Work out the finished part from the listing and answer in its coordinate system (mm). A direction names the side the tool comes from. Round coordinates to 2 decimals unless told otherwise and drop trailing zeros. Loops run counter-clockwise (first coordinate to the right, second up) from the corner with the lowest first, then second, coordinate; pieces in that order, holes last. Notation, with made-up numbers: (81.25, 17) -> (117.25, 17) arc R8 ccw to (117.25, 27) -> close; hole circle Ø7 at (-19.75, 47). An arc over 180 degrees is marked (long way). Use one line per item in the form item = value.
```python
from build123d import *

# Parameters (mm, degrees)
SKETCH2_R           = 1.95
SKETCH2_R_2         = 12.5
BOSS_EXTRUDE1_DEPTH = 3.175


with BuildPart() as part:
    # Sketch2 → Boss-Extrude1 (new body)
    with BuildSketch(Plane.XY):
        Polygon((-3.175, 0), (66.675, 0), (66.675, 12.7), (63.5, 12.7), (63.5, 14.375), (60.412, 14.375), (60.412, 12.625), (57.912, 12.625), (57.912, 14.375), (57.15, 14.375), (57.15, 17.375), (57.912, 17.375), (57.912, 19.125), (60.412, 19.125), (60.412, 17.375), (63.5, 17.375), (63.5, 27.075), (60.412, 27.075), (60.412, 25.325), (57.912, 25.325), (57.912, 27.075), (57.15, 27.075), (57.15, 30.075), (57.912, 30.075), (57.912, 31.825), (60.412, 31.825), (60.412, 30.075), (63.5, 30.075), (63.5, 31.75), (66.675, 31.75), (66.675, 44.45), (-3.175, 44.45), (-3.175, 31.75), (0, 31.75), (0, 30.075), (3.088, 30.075), (3.088, 31.825), (5.588, 31.825), (5.588, 30.075), (6.35, 30.075), (6.35, 27.075), (5.588, 27.075), (5.588, 25.325), (3.088, 25.325), (3.088, 27.075), (0, 27.075), (0, 17.375), (3.088, 17.375), (3.088, 19.125), (5.588, 19.125), (5.588, 17.375), (6.35, 17.375), (6.35, 14.375), (5.588, 14.375), (5.588, 12.625), (3.088, 12.625), (3.088, 14.375), (0, 14.375), (0, 12.7), (-3.175, 12.7), align=None)
        with Locations((16.25, 6.725)):
            Circle(SKETCH2_R, mode=Mode.SUBTRACT)
        with Locations((47.25, 6.725)):
            Circle(SKETCH2_R, mode=Mode.SUBTRACT)
        with Locations((16.25, 37.725)):
            Circle(SKETCH2_R, mode=Mode.SUBTRACT)
        with Locations((31.75, 22.225)):
            Circle(SKETCH2_R_2, mode=Mode.SUBTRACT)
        with Locations((47.25, 37.725)):
            Circle(SKETCH2_R, mode=Mode.SUBTRACT)
    extrude(amount=BOSS_EXTRUDE1_DEPTH)


solid = part.part
```
(1) For a pull along X with two mould halves and no side action, classify faces 1 (the flat face through (6.35, 16, 2)), 2 (the flat face through (3.088, 13, 2)), 3 (the flat face through (2, 30.075, 2)), 4 (the flat face through (63.5, 22, 2)) as +X half, -X half, draft (parallel to the pull), parting line (faces both ways), or undercut.
Completed:
face_1 = -X half
face_2 = undercut
face_3 = draft
face_4 = +X half
(2) For faces 5 (the flat face through (2, 17.375, 2)), 6 (the flat face through (32, 44.45, 2)), 7 (the flat face through (62, 27.075, 2)), 8 (the flat face through (3.088, 26, 2)), determine the directions among +Z, -Z, +X, -X, +Y, -Y from which every point of the face is accessible in a straight line to the end or side of a thin tool.
Completed:
face_5 = +Z, -Z, -X
face_6 = +Z, -Z, +X, -X, +Y
face_7 = +Z, -Z, +X
face_8 = +Z, -Z
(3) Find section D-D, the plane y = 24.5. Write down the section's boundary in (x, z) (3 decimals), then the cut area to 3 significant figures.
Completed:
outline = (0, 0) -> (19.459, 0) -> (19.459, 3.175) -> (0, 3.175) -> close; (44.041, 0) -> (63.5, 0) -> (63.5, 3.175) -> (44.041, 3.175) -> close
area = 124 mm2
(4) Find section B-B, the plane x = 31.75. Write down the section's boundary in (y, z) (3 decimals).
Completed:
outline = (0, 0) -> (9.725, 0) -> (9.725, 3.175) -> (0, 3.175) -> close; (34.725, 0) -> (44.45, 0) -> (44.45, 3.175) -> (34.725, 3.175) -> close
(5) Find section C-C, the plane y = 7.5. Write down the section's boundary in (x, z) (3 decimals).
Completed:
outline = (-3.175, 0) -> (14.461, 0) -> (14.461, 3.175) -> (-3.175, 3.175) -> close; (18.039, 0) -> (45.461, 0) -> (45.461, 3.175) -> (18.039, 3.175) -> close; (49.039, 0) -> (66.675, 0) -> (66.675, 3.175) -> (49.039, 3.175) -> close
(6) Consider L1, parallel to Y at x = 47.25, z = 1.15 (3 decimals); L2, parallel to Y at x = 1, z = 2 (3 decimals); L3, parallel to X at y = 22.5, z = 0.3. Determine where each line is inside the solid, lowest interval first.
Completed:
L1 = 0 to 4.775, 8.675 to 35.775, 39.675 to 44.45
L2 = 0 to 14.375, 17.375 to 27.075, 30.075 to 44.45
L3 = 0 to 19.25, 44.25 to 63.5
(7) Find section A-A, the plane x = 16.25. Write down the section's boundary in (y, z) (3 decimals).
Completed:
outline = (0, 0) -> (4.775, 0) -> (4.775, 3.175) -> (0, 3.175) -> close; (8.675, 0) -> (35.775, 0) -> (35.775, 3.175) -> (8.675, 3.175) -> close; (39.675, 0) -> (44.45, 0) -> (44.45, 3.175) -> (39.675, 3.175) -> close
(8) Given P1, Ø1.4, axis at y = 18, z = 1, coming from the -X side; P2, Ø1.4, axis at y = 31, z = 1.5, coming from the +X side, each flat-ended and moving along its own axis, determine where each tip first touches the part or whether it passes through.
Completed:
P1 = 0
P2 = 63.5
